Here's how the part is built. I have some questions about the finished solid (model axes, mm). A direction names the side the tool comes from. Coordinates: 2 decimals unless noted, no trailing zeros. Write each loop counter-clockwise with the first axis right and the second up, starting at its lowest first coordinate (ties: lowest second). Pieces come first, ordered by that corner, then holes.
(1) Imagine slicing it at C-C, the plane y = 19.5. List the corners of the cut face in (x, z) for me, plus the area to 3 significant figures.
(2) Thinking about a two-plate mould opening in Z: for faces 6 (the cylindrical face through (29.43, 36.6, -25.03)), 7 (the flat face through (30, 18, -43)), 8 (the flat face through (25, 2, 0)), 9 (the cylindrical face through (12.154, 1.972, -61.497)), which applies, released by +Z, released by -Z, zero draft, split by the parting line, or undercut?
(3) Imagine slicing it at B-B, the plane z = -20. List the corners of the cut face in (x, y) for me, plus the area to 3 significant figures.
(4) For pin 1 Ø6 at (x, y) = (33, 40) entering from -Z; pin 2 Ø5 at (x, y) = (41.5, 10.5) entering from +Z; pin 3 Ø1.2 at (x, z) = (20.5, -26) entering from +Y; pin 4 Ø12 at (x, z) = (48, -52.5) entering from -Y, each with a flat end and sliding along its axis, tell me the tip position at first contact or that it passes through.
(5) Please list where these lines run through material, in increasing order: probe 1 along Y at (x, z) = (12, -22.5); probe 2 along Z at (x, y) = (35, 47.5); probe 3 along Y at (x, z) = (12, -41).
(6) Imagine slicing it at A-A, the plane z = -58. List the corners of the cut face in (x, y) for me, plus the area to 3 significant figures.
(7) Which directions (+Z, -Z, +X, -X, +Y, -Y) give clear straight access to the entire face, cutting with the end or side of a thin tool? Please do faces 1 (the flat face through (49, 39, -25)), 2 (the flat face through (40, 37, -44)), 3 (the flat face through (28, 4, -33)), 4 (the flat face through (8, 27, -22)), 5 (the flat face through (8, 19, -44)).
(8) Imagine slicing it at D-D, the plane x = 38. State how many separate pieces and enclosed holes the cut face has, plus the area to 3 significant figures.
```python
from build123d import *
from build123d.topology import SkipClean

# Parameters (mm, degrees)
SKETCH1_R               = 3.5
SKETCH1_W               = 56
SKETCH1_H               = 4
SKETCH1_H_2             = 12
BOSS_EXTRUDE1_DEPTH     = 4
SKETCH1_3_W             = 56
SKETCH1_3_H             = 4
BOSS_EXTRUDE2_DEPTH     = 36
SKETCH2_R               = 5
CUT_EXTRUDE1_DEPTH      = 36
BOSS_EXTRUDE3_START     = -20
BOSS_EXTRUDE3_OUTLINE_R = 9.5
BOSS_EXTRUDE3_DEPTH     = 20
CUT_EXTRUDE2_START      = -21
SKETCH2_4_R             = 4
CUT_EXTRUDE2_DEPTH      = 21
SKETCH4_W               = 61
SKETCH4_H               = 12
CUT_EXTRUDE3_DEPTH      = 47
BOSS_EXTRUDE4_START     = 1
SKETCH5_R               = 4
SKETCH5_R_2             = 9.5
SKETCH5_R_3             = 5
BOSS_EXTRUDE4_DEPTH     = 1
BOSS_EXTRUDE5_START     = 8
BOSS_EXTRUDE5_DEPTH     = 8
BOSS_EXTRUDE6_DEPTH     = 8
SKETCH2_6_R             = 9.5
SKETCH2_6_R_2           = 5
SKETCH2_6_R_3           = 4
BOSS_EXTRUDE7_DEPTH     = 1


# Read off the part's stored shape, not the designer's step: Boss-Extrude3
with BuildPart() as part:
    # Sketch1 → Boss-Extrude1 (new body)
    # profile 1 of 5: a face of its own
    with BuildSketch(Plane(origin=(0, 0, 0), x_dir=(1, 0, 0), z_dir=(0, 1, 0))):
        Polygon((56, 23), (0, 23), (0, 10), (10, 0), (40, 0), (56, 16), align=None)
        with Locations(Location((10, 8, 0), (0, 0, 270))):
            Circle(SKETCH1_R, mode=Mode.SUBTRACT)
        with Locations(Location((37, 8, 0), (0, 0, 270))):
            Circle(SKETCH1_R, mode=Mode.SUBTRACT)
    # profile 2 of 5: a face of its own
    with BuildSketch(Plane(origin=(0, 0, 0), x_dir=(1, 0, 0), z_dir=(0, 1, 0))):
        with Locations((28, 25)):
            Rectangle(SKETCH1_W, SKETCH1_H)
    # profile 3 of 5: a face of its own
    with BuildSketch(Plane(origin=(0, 0, 0), x_dir=(1, 0, 0), z_dir=(0, 1, 0))):
        with Locations((28, 33)):
            Rectangle(SKETCH1_W, SKETCH1_H_2)
    # profile 4 of 5: a face of its own
    with BuildSketch(Plane(origin=(0, 0, 0), x_dir=(1, 0, 0), z_dir=(0, 1, 0))):
        with Locations((28, 41)):
            Rectangle(SKETCH1_W, SKETCH1_H)
    # profile 5 of 5: a face of its own
    with BuildSketch(Plane(origin=(0, 0, 0), x_dir=(1, 0, 0), z_dir=(0, 1, 0))):
        Polygon((40, 66), (10, 66), (0, 56), (0, 43), (56, 43), (56, 50), align=None)
        with Locations(Location((12, 58, 0), (0, 0, 270))):
            Circle(SKETCH1_R, mode=Mode.SUBTRACT)
        with Locations(Location((39, 58, 0), (0, 0, 270))):
            Circle(SKETCH1_R, mode=Mode.SUBTRACT)
    extrude(amount=BOSS_EXTRUDE1_DEPTH)

    # Sketch1<3> → Boss-Extrude2 (add)
    with BuildSketch(Plane(origin=(0, 0, 0), x_dir=(1, 0, 0), z_dir=(0, 1, 0))):
        with Locations((28, 41)):
            Rectangle(SKETCH1_3_W, SKETCH1_3_H)
        with Locations((28, 25)):
            Rectangle(SKETCH1_3_W, SKETCH1_3_H)
    extrude(amount=BOSS_EXTRUDE2_DEPTH)

    # Sketch2 → Cut-Extrude1 (cut)
    with BuildSketch(Plane.XY.offset(-23)):
        with Locations((12, 23)):
            Circle(SKETCH2_R)
    extrude(amount=-CUT_EXTRUDE1_DEPTH, mode=Mode.SUBTRACT)

    # Boss-Extrude3 outline → Boss-Extrude3 (add)
    with BuildSketch(Plane.XY.offset(-23).offset(BOSS_EXTRUDE3_START)):
        with BuildLine():
            Line((28, 36), (2, 36))
            ThreePointArc((2, 36), (0.585786438, 35.414213562), (0, 34))
            Line((0, 34), (0, 4))
            Line((0, 4), (56, 4))
            Line((56, 4), (60.615384615, 15.076923077))
            ThreePointArc((60.615384615, 15.076923077), (60.160251472, 19.773500981), (56, 22))
            Line((56, 22), (49, 36))
            Line((49, 36), (49, 41.5))
            ThreePointArc((49, 41.5), (39.5, 51), (30, 41.5))
            Line((30, 41.5), (30, 38))
            ThreePointArc((30, 38), (29.414213562, 36.585786438), (28, 36))
        make_face()
        with Locations((12, 23)):
            Circle(BOSS_EXTRUDE3_OUTLINE_R, mode=Mode.SUBTRACT)
    extrude(amount=BOSS_EXTRUDE3_DEPTH)

    # Sketch2<4> → Cut-Extrude2 (cut)
    with SkipClean():  # the faces are left unmerged after this step: merging them gives an invalid solid
        with BuildSketch(Plane.XY.offset(-23).offset(CUT_EXTRUDE2_START)):
            with BuildLine():
                Line((30, 38), (30, 41.5))
                ThreePointArc((30, 41.5), (39.5, 51), (49, 41.5))
                Line((49, 41.5), (49, 36))
                Line((49, 36), (56, 36))
                Line((56, 36), (56, 22))
                ThreePointArc((56, 22), (59.535533906, 20.535533906), (61, 17))
                ThreePointArc((61, 17), (60.902903378, 16.019419324), (60.615384615, 15.076923077))
                Line((60.615384615, 15.076923077), (56, 4))
                Line((56, 4), (64.674649384, 4))
                Line((64.674649384, 4), (64.674649384, 61.803942061))
                Line((64.674649384, 61.803942061), (-6.186238706, 61.803942061))
                Line((-6.186238706, 61.803942061), (-6.186238706, 4))
                Line((-6.186238706, 4), (0, 4))
                Line((0, 4), (0, 34))
                Line((0, 34), (0, 36))
                Line((0, 36), (2, 36))
                Line((2, 36), (28, 36))
                ThreePointArc((28, 36), (29.414213562, 36.585786438), (30, 38))
            make_face()
            with BuildLine():
                ThreePointArc((0, 34), (0.585786438, 35.414213562), (2, 36))
                Line((2, 36), (0, 36))
                Line((0, 36), (0, 34))
            make_face()
            Polygon((56, 36), (49, 36), (56, 22), align=None)
            with Locations((39.5, 41.5)):
                Circle(SKETCH2_4_R)
        extrude(amount=CUT_EXTRUDE2_DEPTH, mode=Mode.SUBTRACT)
    add(part.part.scale(1), mode=Mode.REPLACE)  # the faces are merged on a copy

    # Sketch4 → Cut-Extrude3 (cut)
    with BuildSketch(Plane(origin=(0, 51, 0), x_dir=(1, 0, 0), z_dir=(0, 1, 0))):
        with Locations((30.5, 33)):
            Rectangle(SKETCH4_W, SKETCH4_H)
    extrude(amount=-CUT_EXTRUDE3_DEPTH, mode=Mode.SUBTRACT)

    # Sketch5 → Boss-Extrude4 (add)
    # profile 1 of 2: a face of its own
    with SkipClean():  # the faces are left unmerged after this step: merging them gives an invalid solid
        with BuildSketch(Plane(origin=(0, 0, -43), x_dir=(-1, 0, 0), z_dir=(0, 0, -1)).offset(BOSS_EXTRUDE4_START)):
            with BuildLine():
                ThreePointArc((-49, 41.5), (-39.5, 32), (-30, 41.5))
                ThreePointArc((-30, 41.5), (-39.5, 51), (-49, 41.5))
            make_face()
            with Locations((-39.5, 41.5)):
                Circle(SKETCH5_R, mode=Mode.SUBTRACT)
        # profile 2 of 2: a face of its own
        with BuildSketch(Plane(origin=(0, 0, -43), x_dir=(-1, 0, 0), z_dir=(0, 0, -1)).offset(BOSS_EXTRUDE4_START)):
            with Locations((-12, 23)):
                Circle(SKETCH5_R_2)
            with Locations(Location((-12, 23, 0), (0, 0, 180))):
                Circle(SKETCH5_R_3, mode=Mode.SUBTRACT)
        extrude(amount=-BOSS_EXTRUDE4_DEPTH)

    # Sketch5<3> → Boss-Extrude5 (add)
    with SkipClean():  # the faces are left unmerged after this step: merging them gives an invalid solid
        with BuildSketch(Plane(origin=(0, 0, -43), x_dir=(-1, 0, 0), z_dir=(0, 0, -1)).offset(BOSS_EXTRUDE5_START)):
            with BuildLine():
                ThreePointArc((-60.615384615, 15.076923077), (-55.019419324, 12.097096622), (-51, 17))
                ThreePointArc((-51, 17), (-52.464466094, 20.535533906), (-56, 22))
                ThreePointArc((-56, 22), (-60.160251472, 19.773500981), (-60.615384615, 15.076923077))
            make_face()
        extrude(amount=-BOSS_EXTRUDE5_DEPTH)

    # Sketch2<5> → Boss-Extrude6 (add)
    with SkipClean():  # the faces are left unmerged after this step: merging them gives an invalid solid
        with BuildSketch(Plane.XY.offset(-23)):
            with BuildLine():
                Line((56, 12), (56, 22))
                ThreePointArc((56, 22), (51, 17), (56, 12))
            make_face()
            with BuildLine():
                ThreePointArc((61, 17), (59.535533906, 20.535533906), (56, 22))
                Line((56, 22), (56, 12))
                ThreePointArc((56, 12), (58.773500981, 12.839748528), (60.615384615, 15.076923077))
                ThreePointArc((60.615384615, 15.076923077), (60.902903378, 16.019419324), (61, 17))
            make_face()
        extrude(amount=BOSS_EXTRUDE6_DEPTH)

    # Sketch2<6> → Boss-Extrude7 (add)
    # profile 1 of 3: a face of its own
    with BuildSketch(Plane.XY.offset(-23)):
        with Locations(Location((12, 23, 0), (0, 0, 180))):
            Circle(SKETCH2_6_R)
        with Locations((12, 23)):
            Circle(SKETCH2_6_R_2, mode=Mode.SUBTRACT)
    # profile 2 of 3: a face of its own
    with BuildSketch(Plane.XY.offset(-23)):
        with BuildLine():
            ThreePointArc((49, 41.5), (39.5, 51), (30, 41.5))
            ThreePointArc((30, 41.5), (30.449124805, 38.613538808), (31.754033308, 36))
            Line((31.754033308, 36), (47.245966692, 36))
            ThreePointArc((47.245966692, 36), (48.550875195, 38.613538808), (49, 41.5))
        make_face()
        with Locations(Location((39.5, 41.5, 0), (0, 0, 180))):
            Circle(SKETCH2_6_R_3, mode=Mode.SUBTRACT)
    # profile 3 of 3: a face of its own
    with BuildSketch(Plane.XY.offset(-23)):
        with BuildLine():
            Line((47.245966692, 36), (31.754033308, 36))
            ThreePointArc((31.754033308, 36), (39.5, 32), (47.245966692, 36))
        make_face()
    extrude(amount=BOSS_EXTRUDE7_DEPTH)


solid = part.part
```
Recorded:
1. outline: (0, -43) - (3.17, -43) - (3.17, -44) - (8.43, -44) - (8.43, -39) - (0, -39) - close; (0, -27) - (8.43, -27) - (8.43, -22) - (3.17, -22) - (3.17, -23) - (0, -23) - close; (15.57, -44) - (20.83, -44) - (20.83, -43) - (51.67, -43) - (51.67, -51) - (60.33, -51) - (60.33, -39) - (15.57, -39) - close; (15.57, -27) - (60.33, -27) - (60.33, -15) - (51.67, -15) - (51.67, -23) - (20.83, -23) - (20.83, -22) - (15.57, -22) - close
1. area: 585 mm2
2. face 6: zero draft
2. face 7: released by -Z
2. face 8: released by +Z
2. face 9: undercut
3. outline: (0, 0) - (56, 0) - (56, 4) - (0, 4) - close; circle Ø10 at (56, 17)
3. area: 303 mm2
4. pin 1: stops at z = -44
4. pin 2: stops at z = -23
4. pin 3: stops at y = 36
4. pin 4: stops at y = 0
5. probe 1: y = 0 to 4, 13.5 to 18, 28 to 32.5
5. probe 2: z = -44 to -39, -27 to -22
5. probe 3: y = 0 to 18, 28 to 36
6. outline: (2, 0) - (8.5, 0) - (8.5, 4) - (2, 4) - close; (15.5, 0) - (35.5, 0) - (35.5, 4) - (15.5, 4) - close; (42.5, 0) - (48, 0) - (48, 4) - (42.5, 4) - close
6. area: 128 mm2
7. face 1: +Z, -Z, +X, +Y
7. face 2: -Z, +X, -X, +Y
7. face 3: +X, -X, +Y
7. face 4: +Z, -X, +Y
7. face 5: -Z, -X, +Y
8. separate pieces: 5
8. enclosed holes: 0
8. area: 549 mm2
